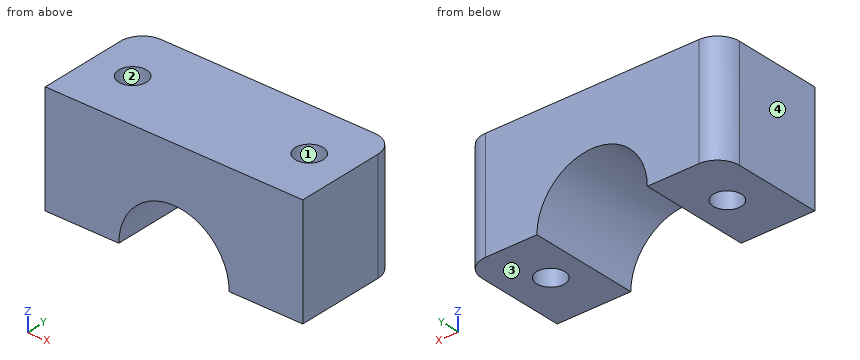
```python
from build123d import *

# Parameters (mm, degrees)
SKETCH1_W           = 35
SKETCH1_H           = 15
BOSS_EXTRUDE1_DEPTH = 15
SKETCH2_R           = 1.9
CUT_EXTRUDE1_DEPTH  = 15
FILLET1_R           = 3
SKETCH3_R           = 7.5
CUT_EXTRUDE2_DEPTH  = 16


with BuildPart() as part:
    # Sketch1 → Boss-Extrude1 (new body)
    with BuildSketch(Plane.XY):
        Rectangle(SKETCH1_W, SKETCH1_H)
    extrude(amount=BOSS_EXTRUDE1_DEPTH)

    # Sketch2 → Cut-Extrude1 (cut)
    with BuildSketch(Plane.XY.offset(15)):
        with Locations((-12, 0)):
            Circle(SKETCH2_R)
        with Locations((12, 0)):
            Circle(SKETCH2_R)
    extrude(amount=-CUT_EXTRUDE1_DEPTH, mode=Mode.SUBTRACT)

    # Fillet1
    fillet1_edges = [part.edges().sort_by_distance(p)[0] for p in [
        (-17.5, 7.5, 7.5),
        (17.5, 7.5, 7.5),
    ]]
    fillet(fillet1_edges, radius=FILLET1_R)

    # Sketch3 → Cut-Extrude2 (cut, through all)
    with BuildSketch(Plane(origin=(0, 7.5, 0), x_dir=(1, 0, 0), z_dir=(0, 1, 0))):
        Circle(SKETCH3_R)
    extrude(amount=-CUT_EXTRUDE2_DEPTH, mode=Mode.SUBTRACT)


solid = part.part
```
The listing builds one solid part. Answer for the finished solid, in the listing's coordinates (mm). Face numbers are marked on the shaded views. Coordinates: 2 decimals unless noted, no trailing zeros. Loops run counter-clockwise (first coordinate to the right, second up) from the corner with the lowest first, then second, coordinate; pieces in that order, holes last. Notation, with made-up numbers: M 24,12.5 L 54,12.5 A10 cw 54,25.5 Z; hole C 25.25,-13 d8. An arc over 180 degrees is marked long. Answer as CSV lines item,"result". Start each with the question number.
(1) The part is cut by section D-D (z = 9). Give the vertices of the cut face in (x, y).
(2) Find the intervals of material crossed by L1, parallel to Y at x = 12, z = 7.5; L2, parallel to X at y = -1.25, z = 13; L3, parallel to X at y = 1.5, z = 8, in increasing order. Write a range as [from, to].
(3) The mould has two halves that part along X. Classify the marked faces 1, 2, 3 and 4: pulls with the +X half, pulls with the -X half, needs draft (parallel to the pull), parting line crosses it, or undercut.
(4) The part is cut by section A-A (x = -12). Give the vertices of the cut face in (y, z).
(5) Given pin 1 (2.5 mm diameter, centred on x = 12, y = 0, fed in from +Z), flat-ended and moving along its own axis, determine where the tip first touches the part or whether it passes through.
(6) The part is cut by section C-C (y = 0). Give the vertices of the cut face in (x, z), and give its area (3 significant figures).
(7) The part is cut by section B-B (z = 6). Give the vertices of the cut face in (x, y).
Determined:
1,outline,"M -17.5,-7.5 L 17.5,-7.5 L 17.5,4.5 A3 ccw 14.5,7.5 L -14.5,7.5 A3 ccw -17.5,4.5 Z; hole C -12,0 d3.8; hole C 12,0 d3.8"
2,L1,"[-7.5, -1.9], [1.9, 7.5]"
2,L2,"[-17.5, -13.43], [-10.57, 10.57], [13.43, 17.5]"
2,L3,"[-17.5, -13.17], [-10.83, 10.83], [13.17, 17.5]"
3,face 1,"undercut"
3,face 2,"undercut"
3,face 3,"needs draft"
3,face 4,"pulls with the -X half"
4,outline,"M -7.5,0 L -1.9,0 L -1.9,15 L -7.5,15 Z; M 1.9,0 L 7.5,0 L 7.5,15 L 1.9,15 Z"
5,pin 1,"through"
6,outline,"M -17.5,0 L -13.9,0 L -13.9,15 L -17.5,15 Z; M -10.1,0 L -7.5,0 A7.5 cw 7.5,0 L 10.1,0 L 10.1,15 L -10.1,15 Z; M 13.9,0 L 17.5,0 L 17.5,15 L 13.9,15 Z"
6,area,"323 mm2"
7,outline,"M -17.5,-7.5 L -4.5,-7.5 L -4.5,7.5 L -14.5,7.5 A3 ccw -17.5,4.5 Z; M 4.5,-7.5 L 17.5,-7.5 L 17.5,4.5 A3 ccw 14.5,7.5 L 4.5,7.5 Z; hole C -12,0 d3.8; hole C 12,0 d3.8"
